Input: part model. Units: mm. Frame: model coordinates. A direction names the side the tool comes from. Round coordinates to 2 decimals unless told otherwise and drop trailing zeros. Loops run counter-clockwise (first coordinate to the right, second up) from the corner with the lowest first, then second, coordinate; pieces in that order, holes last. Notation, with made-up numbers: (-2.5, -39.5) -> (49.5, -39.5) arc R27 ccw to (49.5, -15.5) -> close; hole circle Ø11 at (22, 25.5). An arc over 180 degrees is marked (long way). Answer as a JSON object with one key per item and string values.
```python
from build123d import *

# Parameters (mm, degrees)
SKETCH1_W            = 254
SKETCH1_H            = 203.2
BOSS_EXTRUDE2_DEPTH  = 25.4
SKETCH2_W            = 24.638
SKETCH2_H            = 162.814
CUT_EXTRUDE1_DEPTH   = 20.955
SKETCH3_R            = 2.54
CUT_EXTRUDE2_DEPTH   = 162.814
SKETCH4_R            = 6.35
CUT_EXTRUDE3_DEPTH   = 330.708
SKETCH5_R            = 5.842
SKETCH5_R_2          = 3.302
BOSS_EXTRUDE3_DEPTH  = 25.4
SKETCH7_R            = 5.842
SKETCH7_R_2          = 3.302
BOSS_EXTRUDE4_DEPTH  = 25.4
SKETCH9_R            = 5.842
SKETCH9_R_2          = 3.302
BOSS_EXTRUDE5_DEPTH  = 73.025
SKETCH11_R           = 6.35
CUT_EXTRUDE4_DEPTH   = 271.907
SKETCH12_R           = 5.842
SKETCH12_R_2         = 3.302
BOSS_EXTRUDE6_DEPTH  = 25.4
SKETCH14_R           = 5.842
SKETCH14_R_2         = 3.302
BOSS_EXTRUDE7_DEPTH  = 73.025
SKETCH17_R           = 5.842
SKETCH17_R_2         = 3.302
BOSS_EXTRUDE8_DEPTH  = 25.4
CUT_EXTRUDE5_DEPTH   = 12.7
SKETCH20_RX          = 44.45
SKETCH20_RY          = 21.59
SKETCH20_RX_2        = 14.8082
SKETCH20_RY_2        = 6.35
CUT_EXTRUDE6_DEPTH   = 20.32
SKETCH24_R           = 2.54
BOSS_EXTRUDE9_DEPTH  = 5.08
SKETCH25_R           = 2.54
BOSS_EXTRUDE10_DEPTH = 5.08
SKETCH28_R           = 6.35
BOSS_EXTRUDE11_DEPTH = 12.7
SKETCH30_R           = 6.35
BOSS_EXTRUDE12_DEPTH = 12.7
SKETCH31_R           = 3.81
CUT_EXTRUDE7_DEPTH   = 150.114
FILLET1_R            = 5.08


with BuildPart() as part:
    # Sketch1 → Boss-Extrude2 (new body)
    with BuildSketch(Plane(origin=(0, 0, 0), x_dir=(1, 0, 0), z_dir=(0, 1, 0))):
        with Locations((127, 101.6)):
            Rectangle(SKETCH1_W, SKETCH1_H)
    extrude(amount=BOSS_EXTRUDE2_DEPTH)

    # Sketch2 → Cut-Extrude1 (cut)
    with BuildSketch(Plane(origin=(0, 25.4, 0), x_dir=(1, 0, 0), z_dir=(0, 1, 0))):
        with Locations((84.709, 101.6)):
            Rectangle(SKETCH2_W, SKETCH2_H)
        with Locations((116.967, 101.6)):
            Rectangle(SKETCH2_W, SKETCH2_H)
        with Locations((149.225, 101.6)):
            Rectangle(SKETCH2_W, SKETCH2_H)
        with Locations((181.483, 101.6)):
            Rectangle(SKETCH2_W, SKETCH2_H)
        with Locations((213.741, 101.6)):
            Rectangle(SKETCH2_W, SKETCH2_H)
    extrude(amount=-CUT_EXTRUDE1_DEPTH, mode=Mode.SUBTRACT)

    # Sketch3 → Cut-Extrude2 (cut)
    with BuildSketch(Plane.XY.offset(-183.007)):
        with Locations((72.39, 25.4)):
            Circle(SKETCH3_R)
        with Locations((104.648, 25.4)):
            Circle(SKETCH3_R)
        with Locations((136.906, 25.4)):
            Circle(SKETCH3_R)
        with Locations((169.164, 25.4)):
            Circle(SKETCH3_R)
        with Locations((201.422, 25.4)):
            Circle(SKETCH3_R)
    extrude(amount=CUT_EXTRUDE2_DEPTH, mode=Mode.SUBTRACT)

    # Sketch4 → Cut-Extrude3 (cut)
    with BuildSketch(Plane(origin=(254, 0, 0), x_dir=(0, 0, -1), z_dir=(1, 0, 0))):
        with Locations((0, 25.4)):
            Circle(SKETCH4_R)
    extrude(amount=-CUT_EXTRUDE3_DEPTH, mode=Mode.SUBTRACT)

    # Sketch5 → Boss-Extrude3 (add)
    with BuildSketch(Plane(origin=(254, 0, 0), x_dir=(0, 0, -1), z_dir=(1, 0, 0))):
        with BuildLine():
            ThreePointArc((5.842, 25.4), (4.130917816, 21.269082184), (0, 19.558))
            Line((0, 19.558), (0, 19.05))
            ThreePointArc((0, 19.05), (4.490128061, 20.909871939), (6.35, 25.4))
            Line((6.35, 25.4), (5.842, 25.4))
        make_face()
        with Locations((0, 25.4)):
            Circle(SKETCH5_R)
        with Locations((0, 25.4)):
            Circle(SKETCH5_R_2, mode=Mode.SUBTRACT)
    extrude(amount=-BOSS_EXTRUDE3_DEPTH)

    # Sketch7 → Boss-Extrude4 (add)
    with BuildSketch(Plane.ZY.offset(-26.67)):
        with BuildLine():
            ThreePointArc((0, 19.558), (-4.130917816, 21.269082184), (-5.842, 25.4))
            Line((-5.842, 25.4), (-6.902928933, 25.4))
            Line((-6.902928933, 25.4), (-6.372464466, 22.098))
            Line((-6.372464466, 22.098), (-4.097007923, 19.395027099))
            Line((-4.097007923, 19.395027099), (0, 18.4548232))
            Line((0, 18.4548232), (0, 19.558))
        make_face()
        with Locations((0, 25.4)):
            Circle(SKETCH7_R)
        with Locations((0, 25.4)):
            Circle(SKETCH7_R_2, mode=Mode.SUBTRACT)
    extrude(amount=-BOSS_EXTRUDE4_DEPTH)

    # Sketch9 → Boss-Extrude5 (add)
    with BuildSketch(Plane(origin=(200.66, 0, 0), x_dir=(0, 0, -1), z_dir=(1, 0, 0))):
        with BuildLine():
            Line((7.296114835, 25.4), (5.842, 25.4))
            ThreePointArc((5.842, 25.4), (4.130917816, 21.269082184), (0, 19.558))
            Line((0, 19.558), (0, 18.462733019))
            Line((0, 18.462733019), (2.519044433, 18.922066711))
            Line((2.519044433, 18.922066711), (5.842, 20.162267681))
            Line((5.842, 20.162267681), (7.296114835, 25.4))
        make_face()
        with Locations((0, 25.4)):
            Circle(SKETCH9_R)
        with Locations((0, 25.4)):
            Circle(SKETCH9_R_2, mode=Mode.SUBTRACT)
    extrude(amount=-BOSS_EXTRUDE5_DEPTH)

    # Sketch11 → Cut-Extrude4 (cut)
    with BuildSketch(Plane(origin=(254, 0, 0), x_dir=(0, 0, -1), z_dir=(1, 0, 0))):
        Circle(SKETCH11_R)
    extrude(amount=-CUT_EXTRUDE4_DEPTH, mode=Mode.SUBTRACT)

    # Sketch12 → Boss-Extrude6 (add)
    with BuildSketch(Plane.ZY):
        with BuildLine():
            ThreePointArc((-5.842, 0), (-4.130917816, 4.130917816), (0, 5.842))
            Line((0, 5.842), (0, 6.35))
            ThreePointArc((0, 6.35), (-4.490128061, 4.490128061), (-6.35, 0))
            Line((-6.35, 0), (-5.842, 0))
        make_face()
        Circle(SKETCH12_R)
        Circle(SKETCH12_R_2, mode=Mode.SUBTRACT)
    extrude(amount=-BOSS_EXTRUDE6_DEPTH)

    # Sketch14 → Boss-Extrude7 (add)
    with BuildSketch(Plane.ZY.offset(-53.34)):
        with BuildLine():
            ThreePointArc((-5.842, 0), (-4.130917816, 4.130917816), (0, 5.842))
            Line((0, 5.842), (0, 7.34197102))
            Line((0, 7.34197102), (-6.416971857, 5.34789306))
            Line((-6.416971857, 5.34789306), (-7.97079884, 0))
            Line((-7.97079884, 0), (-5.842, 0))
        make_face()
        Circle(SKETCH14_R)
        Circle(SKETCH14_R_2, mode=Mode.SUBTRACT)
    extrude(amount=-BOSS_EXTRUDE7_DEPTH)

    # Sketch17 → Boss-Extrude8 (add)
    with BuildSketch(Plane(origin=(227.33, 0, 0), x_dir=(0, 0, -1), z_dir=(1, 0, 0))):
        with BuildLine():
            Line((0, 7.437449264), (0, 5.842))
            ThreePointArc((0, 5.842), (4.130917816, 4.130917816), (5.842, 0))
            Line((5.842, 0), (6.728774343, 0))
            Line((6.728774343, 0), (5.842, 4.854950807))
            Line((5.842, 4.854950807), (0, 7.437449264))
        make_face()
        Circle(SKETCH17_R)
        Circle(SKETCH17_R_2, mode=Mode.SUBTRACT)
    extrude(amount=-BOSS_EXTRUDE8_DEPTH)

    # Sketch19 → Cut-Extrude5 (cut)
    with BuildSketch(Plane(origin=(0, 25.4, 0), x_dir=(1, 0, 0), z_dir=(0, 1, 0))):
        Polygon((13.97, 90.043), (64.77, 90.043), (64.77, 20.193), (34.29, 20.193), (34.29, 69.723), (13.97, 69.723), align=None)
    extrude(amount=-CUT_EXTRUDE5_DEPTH, mode=Mode.SUBTRACT)

    # Sketch20 → Cut-Extrude6 (cut)
    with BuildSketch(Plane(origin=(0, 25.4, 0), x_dir=(1, 0, 0), z_dir=(0, 1, 0))):
        with Locations(Location((43.18, 142.163874998), (0, 0, -90))):
            Ellipse(SKETCH20_RX, SKETCH20_RY)
        with Locations(Location((43.18, 142.163874998), (0, 0, 90))):
            Ellipse(SKETCH20_RX_2, SKETCH20_RY_2, mode=Mode.SUBTRACT)
    extrude(amount=-CUT_EXTRUDE6_DEPTH, mode=Mode.SUBTRACT)

    # Sketch24 → Boss-Extrude9 (add)
    with BuildSketch(Plane(origin=(0, 25.4, 0), x_dir=(1, 0, 0), z_dir=(0, 1, 0))):
        with Locations((24.13, 44.958)):
            Circle(SKETCH24_R)
        with Locations((234.95, 44.958)):
            Circle(SKETCH24_R)
    extrude(amount=BOSS_EXTRUDE9_DEPTH)

    # Sketch25 → Boss-Extrude10 (add)
    with BuildSketch(Plane(origin=(0, 25.4, 0), x_dir=(1, 0, 0), z_dir=(0, 1, 0))):
        with Locations((43.18, 142.163874998)):
            Circle(SKETCH25_R)
        with Locations((234.95, 142.163874998)):
            Circle(SKETCH25_R)
    extrude(amount=BOSS_EXTRUDE10_DEPTH)

    # Sketch28 → Boss-Extrude11 (add)
    with BuildSketch(Plane(origin=(177.8, 0, 0), x_dir=(0, 0, -1), z_dir=(1, 0, 0))):
        with BuildLine():
            Line((203.2, 19.05), (203.2, 12.7))
            Line((203.2, 12.7), (203.2, 6.35))
            Line((203.2, 6.35), (213.36, 6.35))
            ThreePointArc((213.36, 6.35), (207.01, 12.7), (213.36, 19.05))
            Line((213.36, 19.05), (203.2, 19.05))
        make_face()
        with Locations((213.36, 12.7)):
            Circle(SKETCH28_R)
    extrude(amount=BOSS_EXTRUDE11_DEPTH)

    # Sketch30 → Boss-Extrude12 (add)
    with BuildSketch(Plane(origin=(76.2, 0, 0), x_dir=(0, 0, -1), z_dir=(1, 0, 0))):
        with BuildLine():
            Line((213.36, 19.05), (203.2, 19.05))
            Line((203.2, 19.05), (203.2, 6.35))
            Line((203.2, 6.35), (213.36, 6.35))
            ThreePointArc((213.36, 6.35), (207.01, 12.7), (213.36, 19.05))
        make_face()
        with Locations((213.36, 12.7)):
            Circle(SKETCH30_R)
    extrude(amount=-BOSS_EXTRUDE12_DEPTH)

    # Sketch31 → Cut-Extrude7 (cut)
    with BuildSketch(Plane(origin=(190.5, 0, 0), x_dir=(0, 0, -1), z_dir=(1, 0, 0))):
        with Locations((213.36, 12.7)):
            Circle(SKETCH31_R)
    extrude(amount=-CUT_EXTRUDE7_DEPTH, mode=Mode.SUBTRACT)

    # Fillet1
    fillet1_edges = [part.edges().sort_by_distance(p)[0] for p in [
        (184.15, 6.35, -203.2),
        (184.15, 19.05, -203.2),
        (69.85, 6.35, -203.2),
        (69.85, 19.05, -203.2),
    ]]
    fillet(fillet1_edges, radius=FILLET1_R)

    # Sketch34 → Revolve1 (revolve)
    with BuildSketch(Plane(origin=(0, 0, -142.163874998), x_dir=(-1, 0, 0), z_dir=(0, 0, -1))):
        Polygon((-234.95, 24.13), (-234.95, 36.83), (-240.03, 36.83), (-237.49, 30.48), (-240.03, 24.13), align=None)
    revolve(axis=Axis((234.95, 24.13, -142.163874998), (0, 1, 0)))

    # Sketch35 → Revolve2 (revolve)
    with BuildSketch(Plane(origin=(0, 0, -142.163874998), x_dir=(-1, 0, 0), z_dir=(0, 0, -1))):
        Polygon((-43.18, 24.13), (-43.18, 36.83), (-38.1, 36.83), (-40.64, 30.48), (-38.1, 24.13), align=None)
    revolve(axis=Axis((43.18, 24.13, -142.163874998), (0, 1, 0)))

    # Sketch38 → Revolve3 (revolve)
    with BuildSketch(Plane(origin=(0, 0, -44.958), x_dir=(-1, 0, 0), z_dir=(0, 0, -1))):
        Polygon((-232.41, 30.48), (-229.87, 36.83), (-234.95, 36.83), (-234.95, 24.13), (-229.87, 24.13), align=None)
    revolve(axis=Axis((234.95, 36.83, -44.958), (0, -1, 0)))

    # Sketch39 → Revolve7 (revolve)
    with BuildSketch(Plane(origin=(0, 0, -44.958), x_dir=(-1, 0, 0), z_dir=(0, 0, -1))):
        Polygon((-24.13, 24.13), (-24.13, 36.83), (-19.05, 36.83), (-21.59, 30.48), (-19.05, 24.13), align=None)
    revolve(axis=Axis((24.13, 24.13, -44.958), (0, 1, 0)))


solid = part.part
```
1) Reachability of faces 1 (the face through (148, 15, -20.193)), 2 (the face through (237.925, 29.033, -143.101)), 3 (the face through (227.33, 2, -3)) from +Z, -Z, +X, -X, +Y, -Y: full face, straight path, thin tool, end or side. Return the list, or none.
Output:
{"face 1": "+Y", "face 2": "none", "face 3": "+Z, +X, -Y"}
2) Section A-A, the plane x = 223. Output: boundary loops of the cut face in (y, z) (3 decimals), plus the area to 3 significant figures.
Output:
{"outline": "(0, -203.2) -> (25.4, -203.2) -> (25.4, -183.007) -> (4.445, -183.007) -> (4.445, -20.193) -> (25.4, -20.193) -> (25.4, -6.35) arc R6.35 cw to (19.05, 0) -> (5.842, 0) arc R5.842 ccw (long way) to (0, -5.842) -> close; hole circle Ø6.604 at (0, 0)", "area": "1,760 mm^2"}
3) Contact query for flat-ended pins moving along their axis: P1, Ø8.5, axis at y = 12.5, z = -215.5, coming from the -X side; P2, Ø4, axis at x = 67.5, z = -210.5, coming from the +Y side; P3, Ø3.5, axis at y = 26, z = -1, coming from the -X side; P4, Ø8, axis at x = 123, z = -151.5, coming from the +Y side (3 decimals). Output: stop coordinate, or through.
Output:
{"P1": "stops at x = 63.5", "P2": "stops at y = 19.05", "P3": "passes through", "P4": "stops at y = 4.445"}
4) Draft query along Z for faces 4 (the face through (0, 13, -100)), 5 (the face through (21.155, 29.033, -44.021)). Return one class per face: +Z half, -Z half, draft (parallel to the pull), parting line (faces both ways), or undercut.
Output:
{"face 4": "draft", "face 5": "undercut"}
5) Section C-C, the plane z = -13. Output: boundary loops of the cut face in (x, y).
Output:
{"outline": "(0, 0) -> (254, 0) -> (254, 25.4) -> (0, 25.4) -> close"}
6) Ray query, probe 1 along Z at (x, y) = (78, 20); probe 2 along Z at (x, y) = (160.5, 9); probe 3 along Z at (x, y) = (44.5, 7). Return the intervals inside material, ascending.
Output:
{"probe 1": "z = -203.2 to -183.01, -20.19 to -3.34", "probe 2": "z = -203.2 to -183.01, -20.19 to 0", "probe 3": "z = -203.2 to -186.53, -156.65 to -127.68, -97.8 to 0"}
